```python
from build123d import *

# Parameters (mm, degrees)
F0_W      = 58.42
F0_H      = 124.46
F1_DEPTH  = 25.4
F3_DEPTH  = 12.7
F2_W      = 14.9100571871
F2_H      = 16.6536653414
F4_DEPTH  = 25.401
F5_DEPTH  = 25.401
F6_R      = 1.778
F8_DEPTH  = 12.7
F9_R      = 6.600990786
F10_DEPTH = 12.701
F12_W     = 24.9527078122
F12_H     = 45.2845413238
F13_DEPTH = 2.54
F14_W     = 11.3247931004
F14_H     = 17.1568840742
F15_DEPTH = 12.701


with BuildPart() as f1:
    # F0 (on Top) → F1 (new body)
    with BuildSketch(Plane.XY):
        with Locations((-18.5432793882, 2.6247613132)):
            Rectangle(F0_W, F0_H)
    extrude(amount=F1_DEPTH)

    # F2 (on Top) → F3 (cut)
    with BuildSketch(Plane.XY):
        Polygon((-2.9867999256, 36.6561636329), (-31.5876603127, 36.6561636329), (-31.5876603127, -13.3048305288), (-24.3469346315, -13.3048305288), (-9.4368774444, -13.3048305288), (-2.9867999256, -13.3048305288), align=None)
    extrude(amount=F3_DEPTH, mode=Mode.SUBTRACT)

    # F2 (on Top) → F4 (cut, through all)
    with BuildSketch(Plane.XY):
        with Locations((-16.8919060379, -21.6316631995)):
            Rectangle(F2_W, F2_H)
    extrude(amount=F4_DEPTH, mode=Mode.SUBTRACT)

    # F2 (on Top) → F5 (cut, through all)
    with BuildSketch(Plane.XY):
        Polygon((-9.4368774444, -29.9584958702), (-24.3469346315, -29.9584958702), (-31.5876603127, -29.9584958702), (-31.5876603127, -35.0270010531), (-2.9867999256, -35.0270010531), (-2.9867999256, -29.9584958702), align=None)
    extrude(amount=F5_DEPTH, mode=Mode.SUBTRACT)

    # F6
    f6_edges = [f1.edges().sort_by_distance(p)[0] for p in [
        (-2.9868, -35.027001, 12.7),
        (-2.9868, -13.304831, 6.35),
        (-2.9868, -29.958496, 12.7),
        (-2.9868, 36.656164, 6.35),
        (-31.58766, 36.656164, 6.35),
        (-31.58766, -13.304831, 6.35),
        (-31.58766, -29.958496, 12.7),
        (-31.58766, -35.027001, 12.7),
    ]]
    fillet(f6_edges, radius=F6_R)

    # F7 (on face) → F8 (cut)
    with BuildSketch(Plane(origin=(0, 0, 0), x_dir=(1, 0, 0), z_dir=(0, 0, -1))):
        with BuildLine():
            Line((-31.5876603127, -10.9698253981), (-31.5876603127, 9.0240317161))
            ThreePointArc((-31.5876603127, 9.0240317161), (-42.5635968021, -0.972896841), (-31.5876603127, -10.9698253981))
        make_face()
        with BuildLine():
            Line((-2.9867999256, 9.5505814534), (-2.9867999256, -11.675666552))
            ThreePointArc((-2.9867999256, -11.675666552), (7.6263240771, -1.0625425493), (-2.9867999256, 9.5505814534))
        make_face()
    extrude(amount=-F8_DEPTH, mode=Mode.SUBTRACT)

    # F9 (on face) → F10 (cut, through all)
    with BuildSketch(Plane(origin=(0, 0, 12.7), x_dir=(1, 0, 0), z_dir=(0, 0, -1))):
        with Locations((-17.4470897764, -18.4470508248)):
            Circle(F9_R)
    extrude(amount=-F10_DEPTH, mode=Mode.SUBTRACT)

    # F12 (on face) → F13 (cut)
    with BuildSketch(Plane(origin=(0, 0, 12.7), x_dir=(1, 0, 0), z_dir=(0, 0, -1))):
        with Locations((-17.5654711202, -11.2502751872)):
            Rectangle(F12_W, F12_H)
    extrude(amount=-F13_DEPTH, mode=Mode.SUBTRACT)

    # F14 (on face) → F15 (cut, through all)
    with BuildSketch(Plane(origin=(0, 0, 12.7), x_dir=(1, 0, 0), z_dir=(0, 0, -1))):
        with Locations((-17.0887093991, 8.5784420371)):
            Rectangle(F14_W, F14_H)
    extrude(amount=-F15_DEPTH, mode=Mode.SUBTRACT)


solid = f1.part
```
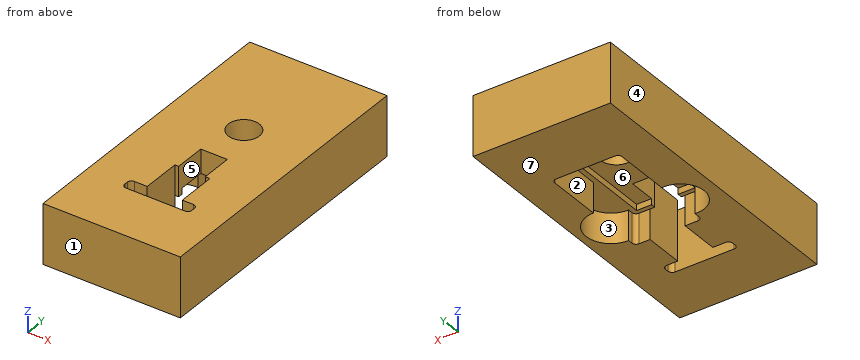
Verification items for the finished model (mm, model axes). Face numbers are marked on the shaded views. A direction names the side the tool comes from. Round coordinates to 2 decimals unless told otherwise and drop trailing zeros. Order: outer loops, then holes, each group sorted by start corner. A loop starts at its lowest first (then second) coordinate and runs counter-clockwise, first axis right, second up.
1) Tool access check on the marked faces 5, 6 and 7. Record the directions out of +Z, -Z, +X, -X, +Y, -Y that give a thin tool (end or side, any length) a straight path to the whole face; none if there is none.
Geometry says:
face 5: +Z, -Z
face 6: -Z
face 7: -Z, +X, -X, +Y, -Y
2) Cross-section at A-A, the plane x = -27. Record the cut outline in (y, z), plus the area to 3 significant figures.
Geometry says:
outline: (-59.61, 0) - (-35.03, 0) - (-35.03, 25.4) - (-59.61, 25.4) - close; (-29.96, 0) - (-13.3, 0) - (-13.3, 12.7) - (-11.39, 12.7) - (-11.39, 15.24) - (33.89, 15.24) - (33.89, 12.7) - (36.66, 12.7) - (36.66, 0) - (64.85, 0) - (64.85, 25.4) - (-29.96, 25.4) - close
area: 2,280 mm2
3) Cross-section at C-C, the plane y = -22. Record the cut outline in (x, z), plus the area to 3 significant figures.
Geometry says:
outline: (-47.75, 0) - (-24.35, 0) - (-24.35, 25.4) - (-47.75, 25.4) - close; (-9.44, 0) - (10.67, 0) - (10.67, 25.4) - (-9.44, 25.4) - close
area: 1,110 mm2
4) Cross-section at B-B, the plane z = 8. Record the cut outline in (x, y).
Geometry says:
outline: (-47.75, -59.61) - (10.67, -59.61) - (10.67, 64.85) - (-47.75, 64.85) - close; hole (-31.59, -33.25) arc R1.78 ccw to (-29.81, -35.03) - (-4.76, -35.03) arc R1.78 ccw to (-2.99, -33.25) - (-2.99, -31.74) arc R1.78 ccw to (-4.76, -29.96) - (-9.44, -29.96) - (-9.44, -13.3) - (-4.76, -13.3) arc R1.78 ccw to (-2.99, -11.53) - (-2.99, -9.55) arc R10.61 ccw to (-2.99, 11.68) - (-2.99, 34.88) arc R1.78 ccw to (-4.76, 36.66) - (-29.81, 36.66) arc R1.78 ccw to (-31.59, 34.88) - (-31.59, 10.97) arc R10.04 ccw (long way) to (-31.59, -9.02) - (-31.59, -11.53) arc R1.78 ccw to (-29.81, -13.3) - (-24.35, -13.3) - (-24.35, -29.96) - (-29.81, -29.96) arc R1.78 ccw to (-31.59, -31.74) - close
5) Depth check by flat-ended pin: pin 1 (8 mm diameter, centred on x = -16.5, y = 13, fed in from -Z). Enter the tip coordinate at first touch or a pass-through.
Geometry says:
pin 1: stops at z = 15.24
6) Draft check along Y on the marked faces 1, 2, 3 and 4. Enter one of: +Y half, -Y half, draft (parallel to the pull), parting line (faces both ways), or undercut.
Geometry says:
face 1: -Y half
face 2: undercut
face 3: undercut
face 4: draft
7) Material ranges on line 1 (Y direction, x = -29.5, z = 11); line 2 (Y direction, x = -17, z = 22.25); line 3 (X direction, y = -1, z = 23.75), recorded low to high.
Geometry says:
line 1: y = -59.61 to -35.03, -29.96 to -13.3, 36.66 to 64.85
line 2: y = -59.61 to -35.03, 0 to 11.86, 25.03 to 64.85
line 3: x = -47.75 to -22.75, -11.43 to 10.67
8) Cross-section at D-D, the plane x = -15. Record the cut outline in (y, z).
Geometry says:
outline: (-59.61, 0) - (-35.03, 0) - (-35.03, 25.4) - (-59.61, 25.4) - close; (0, 15.24) - (12.32, 15.24) - (12.32, 25.4) - (0, 25.4) - close; (24.58, 15.24) - (33.89, 15.24) - (33.89, 12.7) - (36.66, 12.7) - (36.66, 0) - (64.85, 0) - (64.85, 25.4) - (24.58, 25.4) - close
